Geometry check sheet. Reference: the model listing, model coordinates, mm. A direction names the side the tool comes from. Give positions to 0.01 mm unless a question says otherwise; leave off trailing zeros. Write each loop counter-clockwise with the first axis right and the second up, starting at its lowest first coordinate (ties: lowest second). Pieces come first, ordered by that corner, then holes.
(1) Cross-section at A-A (x = -2.5). Record the boundary of the cut face in (y, z), and give its area (3 significant figures).
(2) Cross-section at D-D (z = -107.5). Record the boundary of the cut face in (x, y), and give its area (3 significant figures).
(3) Thickness scan on line 1 along X through (y, z) = (-2.5, -10); line 2 along Z through (x, y) = (-113, -2.2); line 3 along Z through (x, y) = (-10, -3.05). Record the ranges inside material, lowest first.
(4) Cross-section at B-B (z = -47.5). Record the boundary of the cut face in (x, y).
(5) Mould release check, pull along Z, two halves, no side actions. Record for faces 1 (the flat face through (-150, -2, -54)), 2 (the cylindrical face through (-38, -2, -81)), 3 (the flat face through (-74, -2, 0)): +Z half, -Z half, draft (parallel to the pull), parting line (faces both ways), or undercut.
(6) Cross-section at C-C (y = -1.4). Count the separate pieces of the cut face and the enclosed holes in it, and give its area (3 significant figures).
(7) Depth check by flat-ended pin: P1, Ø2.5, axis at x = -2.5, z = -10.5, coming from the +Y side; P2, Ø4, axis at x = -10, z = -2.5, coming from the +Y side; P3, Ø0.9, axis at y = -1.5, z = -76, coming from the +X side. Enter the tip coordinate at first touch or a pass-through.
(8) Tool access check on faces 4 (the cylindrical face through (-2.57, -4.01, -49)), 5 (the flat face through (-75, -3, -29)), 6 (the flat face through (-3, -1, -60)). Record the directions out of +Z, -Z, +X, -X, +Y, -Y that give a thin tool (end or side, any length) a straight path to the whole face; none if there is none.
Autodesk Inventor part; units mm, degrees
ref_plane "YZ Plane" through (0, 0, 0) normal (1, 0, 0) x (0, 1, 0)
ref_plane "XZ Plane" through (0, 0, 0) normal (0, 1, 0) x (-1, 0, 0)
ref_plane "XY Plane" through (0, 0, 0) normal (0, 0, 1) x (1, 0, 0)
sketch "Sketch1" plane through (0, 0, 0) normal (0, 1, 0) x (-1, 0, 0)
  line L0 (0, 0) -> (150, 0)
  line L1 (150, 0) -> (150, -110)
  line L2 (150, -110) -> (0, -110)
  line L3 (0, -110) -> (0, 0)
  line L4 (40, -60) -> (0, -60)
  line L5 (0, -60) -> (0, -102)
  line L6 (0, -102) -> (40, -102)
  line L7 (40, -102) -> (40, -60)
  circle A0 centre (2.5, -62.5) radius 1.5
  circle A1 centre (2.5, -99.5) radius 1.5
  circle A2 centre (34.825, -81) radius 3.175
  circle A3 centre (33.825, -81) radius 3.175
  line L8 (34.825, -77.825) -> (33.825, -77.825)
  line L9 (34.825, -84.175) -> (33.825, -84.175)
  line L10 (37, -77.825) -> (37, -84.175) construction
  line L11 (25, -96) -> (0, -96)
  line L12 (0, -96) -> (0, -66)
  line L13 (0, -66) -> (25, -66)
  line L14 (25, -66) -> (25, -96)
  line L15 (5, -102) -> (5, -96)
  line L16 (5, -66) -> (5, -60)
  line L17 (5, -50) -> (0, -50)
  line L18 (0, -50) -> (0, -8)
  line L19 (0, -8) -> (5, -8)
  line L20 (5, -8) -> (5, -50)
  line L21 (5, -96) -> (5, -66)
  line L22 (80, -50) -> (70, -50)
  line L23 (70, -50) -> (70, -8)
  line L24 (70, -8) -> (80, -8)
  line L25 (80, -8) -> (80, -50)
  point P0 (0, -81)
  point P1 (40, -81)
  point P2 (0, -60)
  point P3 (25, -81)
  point P4 (5, -99)
  point P5 (0, -66)
  point P6 (0, -96)
  point P7 (0, -50)
  point P8 (70, -29)
  point P9 (5, -29)
  dimension "d0" = 110
  dimension "d3" = 42
  dimension "d6" = 40
  dimension "d13" = 3
  dimension "d14" = 3
  dimension "d18" = 2.5
  dimension "d19" = 2.5
  dimension "d20" = 2.5
  dimension "d21" = 2.5
  dimension "d22" = 6.35
  dimension "d23" = 1
  dimension "d26" = 37
  dimension "d29" = 25
  dimension "d30" = 30
  dimension "d31" = 5
  dimension "d32" = 150
  dimension "d33" = 8
  dimension "d34" = 42
  dimension "d35" = 5
  dimension "d36" = 8
  dimension "d73" = 10
  dimension "d74" = 42
  dimension "d75" = 70
extrude "Extrusion1" add sketch "Sketch1" against normal blind 5 contours L0 L1 L2 L3 L6 L7 L4 L17 L20 L19 | L19 L20 L17 L3 | L4 L16 L13 L3 | L3 L11 L15 L6 | L13 L21 L11 L3 | L4 L7 L6 L15 L11 L14 L13 L16 | L13 L14 L11 L21 | A0 | A1 | A2 A3 | A2 A3 L8 | L9 A3 A2 | A3 A2 | A2 A3 | L22 L23 L24 L25
extrude "Extrusion2" cut sketch "Sketch1" against normal blind 5 contours A0 | A1 | A2 A3 | A2 A3 L8 | L9 A3 A2 | A3 A2 | A2 A3
extrude "Extrusion3" cut sketch "Sketch1" against normal blind 3 contours L19 L20 L17 L3 | L4 L16 L13 L3 | L3 L11 L15 L6 | L13 L21 L11 L3 | L22 L23 L24 L25
sketch "Sketch2" plane through (0, -3, 0) normal (0, 1, 0) x (1, 0, 0)
  line L0 (-5, 50) -> (0, 50)
  line L1 (0, 50) -> (0, 8)
  line L2 (0, 8) -> (-5, 8)
  point P0 (0, 0)
  point P1 (-2.5, 47.5)
  point P2 (-2.5, 10.5)
  dimension "d44" = 2.5
  dimension "d45" = 2.5
  dimension "d46" = 2.5
  dimension "d47" = 2.5
hole "Hole1" at (-2.5, -3, -47.5) at (-2.5, -3, -10.5) direction (0, -1, 0) diameter 3 end through all
sketch "Sketch3" plane through (0, 0, 0) normal (0, 1, 0) x (1, 0, 0)
  line L0 (0, 0) -> (0, 8)
  line L1 (-150, 0) -> (0, 0)
  line L2 (0, 110) -> (-150, 110)
  line L3 (0, 102) -> (0, 110)
  point P0 (-10, 2.5)
  point P1 (-10, 107.5)
  dimension "d55" = 10
  dimension "d56" = 2.5
  dimension "d57" = 2.5
  dimension "d58" = 10
hole "Hole2" at (-10, 0, -2.5) at (-10, 0, -107.5) direction (0, -1, 0) diameter 3 depth 6 tip angle 118
pattern_linear "Rectangular Pattern1" count 2 spacing 135 along (-1, 0, 0) of "Hole2"
sketch "Sketch4" plane through (0, -5, 0) normal (0, -1, 0) x (1, 0, 0)
  line L0 (-113, -10) -> (-55, -10) construction
  line L1 (-55, -10) -> (-55, -59) construction
  line L2 (-55, -59) -> (-113, -59) construction
  line L3 (-113, -59) -> (-113, -10) construction
  line L4 (0, 0) -> (-150, 0) construction
  line L5 (0, -110) -> (0, 0) construction
  dimension "d69" = 58
  dimension "d70" = 49
  dimension "d71" = 10
  dimension "d72" = 55
hole "Hole3" at (-113, -5, -10) at (-55, -5, -10) at (-55, -5, -59) at (-113, -5, -59) direction (0, 1, 0) diameter 2.459 end through all
properties part number "Camera plate" material "Aluminum 6061"
Reply:
1. outline: (-5, -110) - (0, -110) - (0, -102) - (-3, -102) - (-3, -101) - (-5, -101) - close; (-5, -98) - (-3, -98) - (-3, -64) - (-5, -64) - close; (-5, -61) - (-3, -61) - (-3, -60) - (0, -60) - (0, -50) - (-3, -50) - (-3, -49) - (-5, -49) - close; (-5, -46) - (-3, -46) - (-3, -12) - (-5, -12) - close; (-5, -9) - (-3, -9) - (-3, -8) - (0, -8) - (0, 0) - (-5, 0) - close
1. area: 274 mm2
2. outline: (-150, -5) - (-146.5, -5) - (-146.5, 0) - (-150, 0) - close; (-143.5, -5) - (-11.5, -5) - (-11.5, 0) - (-143.5, 0) - close; (-8.5, -5) - (0, -5) - (0, 0) - (-8.5, 0) - close
2. area: 720 mm2
3. line 1: x = -150 to -114.23, -111.77 to -80, -70 to -56.23, -53.77 to -5
3. line 2: z = -110 to -60.23, -57.77 to -11.23, -8.77 to 0
3. line 3: z = -110 to -109, -106 to -4, -1 to 0
4. outline: (-150, -5) - (-4, -5) - (-4, -3) - (-5, -3) - (-5, 0) - (-70, 0) - (-70, -3) - (-80, -3) - (-80, 0) - (-150, 0) - close; (-1, -5) - (0, -5) - (0, -3) - (-1, -3) - close
5. face 1: draft
5. face 2: undercut
5. face 3: +Z half
6. separate pieces: 1
6. enclosed holes: 10
6. area: 15,600 mm2
7. P1: passes through
7. P2: stops at y = 0
7. P3: stops at x = -5
8. face 4: +Y, -Y
8. face 5: +Y
8. face 6: +X, +Y
